The listing builds one solid part. Answer for the finished solid, in the listing's coordinates (mm). A direction names the side the tool comes from. Coordinates: 2 decimals unless noted, no trailing zeros. Order: outer loops, then holes, each group sorted by start corner. A loop starts at its lowest first (then second) coordinate and runs counter-clockwise, first axis right, second up. Notation, with made-up numbers: (12, 30.25) - (33, 30.25) arc R20 cw to (33, 40.25) - close; hole circle Ø5 at (62, 4). An arc over 180 degrees is marked (long way). Use a Markdown table: item, result. Add a question column.
Item 1: The part is cut by section A-A, the plane z = -3.25. Give the vertices of the cut face in (x, y), then the cut area to 3 significant figures.
Item 2: The part is cut by section B-B, the plane z = 3. Give the vertices of the cut face in (x, y), then the cut area to 3 significant figures.
Item 3: For faces 1 (the cylindrical face through (-0.931, -1.214, 2.969)), 2 (the cylindrical face through (0.406, 1.288, -0.057)), determine the directions among +Z, -Z, +X, -X, +Y, -Y from which every point of the face is accessible in a straight line to the end or side of a thin tool.
Item 4: Find the intervals of material crossed by line 1 along Y through (x, z) = (-0.05, -0.75); line 2 along Z through (x, y) = (0.9, -0.65); line 3 along Y through (x, z) = (1.05, -1.75), in increasing order.
from build123d import *

# Parameters (mm, degrees)
FILLET1_R = 2
SKETCH2_W = 0.5
SKETCH2_H = 0.029991608
SKETCH3_W = 0.5
SKETCH3_H = 0.05
SKETCH4_W = 0.5
SKETCH4_H = 0.03
SKETCH5_W = 0.5
SKETCH5_H = 0.03


with BuildPart() as part:
    # Sketch1 → Revolve1 (revolve)
    with BuildSketch(Plane(origin=(0, 0, 0), x_dir=(0, 0, -1), z_dir=(1, 0, 0))):
        with BuildLine():
            Line((2.6, 1.5), (3.5, 1.5))
            ThreePointArc((3.5, 1.5), (3.853553391, 1.353553391), (4, 1))
            Line((4, 1), (4, 0))
            Line((4, 0), (-4, 0))
            Line((-4, 0), (-4, 1))
            ThreePointArc((-4, 1), (-3.853553391, 1.353553391), (-3.5, 1.5))
            Line((-3.5, 1.5), (-2.6, 1.5))
            ThreePointArc((-2.6, 1.5), (-2.529289322, 1.470710678), (-2.5, 1.4))
            Line((-2.5, 1.4), (-2.5, 1.3))
            Line((-2.5, 1.3), (2.5, 1.3))
            Line((2.5, 1.3), (2.5, 1.4))
            ThreePointArc((2.5, 1.4), (2.529289322, 1.470710678), (2.6, 1.5))
        make_face()
    revolve(axis=Axis((0, 0, 30.94688027), (0, 0, -1)))

    # Fillet1
    fillet1_edges = [part.edges().sort_by_distance(p)[0] for p in [
        (0, -1.3, -2.5),
        (0, -1.3, 2.5),
    ]]
    fillet(fillet1_edges, radius=FILLET1_R)

    # Sketch2 → Revolve2 (revolve)
    with BuildSketch(Plane(origin=(0, 0, 0), x_dir=(0, 0, -1), z_dir=(1, 0, 0))):
        with Locations((-1.455572809, 1.314995804)):
            Rectangle(SKETCH2_W, SKETCH2_H)
    revolve(axis=Axis((0, 0, 2.184724067), (0, 0, -1)))

    # Sketch3 → Revolve3 (revolve)
    with BuildSketch(Plane(origin=(0, 0, 0), x_dir=(0, 0, -1), z_dir=(1, 0, 0))):
        with Locations((0.053199548, 1.325)):
            Rectangle(SKETCH3_W, SKETCH3_H)
    revolve(axis=Axis((0, 0, 0.48939527), (0, 0, -1)))

    # Sketch4 → Revolve4 (revolve)
    with BuildSketch(Plane(origin=(0, 0, 0), x_dir=(0, 0, -1), z_dir=(1, 0, 0))):
        with Locations((-2.972757668, 1.515)):
            Rectangle(SKETCH4_W, SKETCH4_H)
    revolve(axis=Axis((0, 0, 0.449237838), (0, 0, -1)))

    # Sketch5 → Revolve5 (revolve)
    with BuildSketch(Plane(origin=(0, 0, 0), x_dir=(0, 0, -1), z_dir=(1, 0, 0))):
        with Locations((2.864549609, 1.515)):
            Rectangle(SKETCH5_W, SKETCH5_H)
    revolve(axis=Axis((0, 0, 0.313399994), (0, 0, -1)))


solid = part.part
Solution:
| question | item | result |
|---|---|---|
| 1 | outline | circle Ø3 at (0, 0) |
| 1 | area | 7.07 mm2 |
| 2 | outline | circle Ø3.06 at (0, 0) |
| 2 | area | 7.35 mm2 |
| 3 | face 1 | +Z, -Z |
| 3 | face 2 | none |
| 4 | line 1 | y = -1.3 to 1.3 |
| 4 | line 2 | z = -3.99 to 3.99 |
| 4 | line 3 | y = -0.77 to 0.77 |
